Geometry check sheet. Reference: drawing and pictorial views, mm from the part's lowest x, y, z. A direction names the side the tool comes from. Give positions to 0.01 mm unless a question says otherwise; leave off trailing zeros. Write each loop counter-clockwise with the first axis right and the second up, starting at its lowest first coordinate (ties: lowest second). Pieces come first, ordered by that corner, then holes. Notation, with made-up numbers: (39.5, 41) -> (90.5, 41) arc R16 ccw to (90.5, 54) -> close; hole circle Ø9 at (26, -30). An arc over 180 degrees is marked (long way). Return JSON: item names as keys, results as strings.
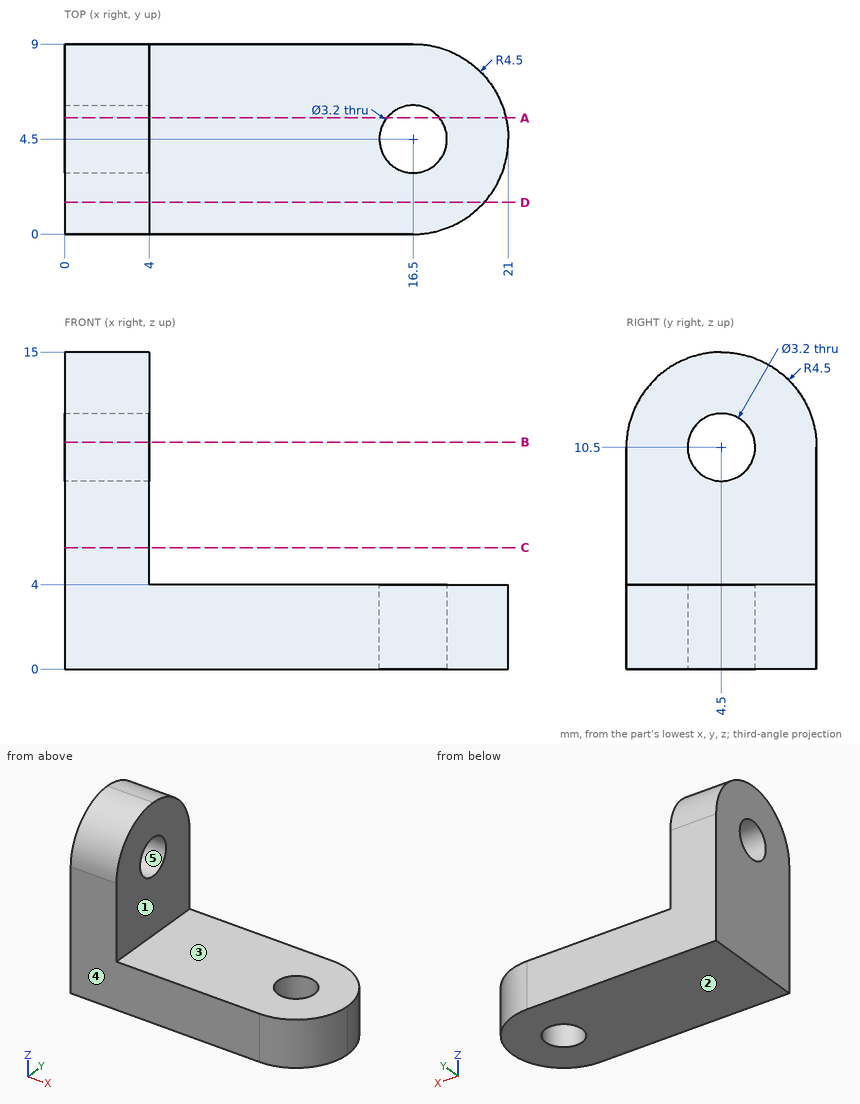
(1) Thickness scan on L1, parallel to Y at x = 2, z = 10.5; L2, parallel to X at y = 4.5, z = 1.45; L3, parallel to X at y = 1, z = 8. Record the ranges inside material, lowest first.
Reply:
{"L1": "0 to 2.9, 6.1 to 9", "L2": "0 to 14.9, 18.1 to 21", "L3": "0 to 4"}
(2) Cross-section at C-C on z = 5.75. Enter the section's corners in (x, y).
Reply:
{"outline": "(0, 0) -> (4, 0) -> (4, 9) -> (0, 9) -> close"}
(3) Cross-section at B-B on z = 10.75. Enter the section's corners in (x, y).
Reply:
{"outline": "(0, 0.01) -> (4, 0.01) -> (4, 2.92) -> (0, 2.92) -> close; (0, 6.08) -> (4, 6.08) -> (4, 8.99) -> (0, 8.99) -> close"}
(4) Set-up check for the marked faces 1 and 2: record each of +Z, -Z, +X, -X, +Y, -Y from which the full face is reachable in a straight line by a thin tool's end or side.
Reply:
{"face 1": "+Z, +X, +Y, -Y", "face 2": "-Z, +X, -X, +Y, -Y"}
(5) Cross-section at D-D on y = 1.5. Enter the section's corners in (x, z).
Reply:
{"outline": "(0, 0) -> (19.85, 0) -> (19.85, 4) -> (4, 4) -> (4, 13.85) -> (0, 13.85) -> close"}
(6) Depth check by flat-ended pin: pin 1 Ø1.5 at (x, z) = (11, 3) entering from -Y; pin 2 Ø3 at (y, z) = (4, 10.5) entering from +X; pin 3 Ø3 at (y, z) = (4.5, 10.5) entering from +X; pin 4 Ø2 at (x, y) = (12, 2) entering from +Z. Enter the tip coordinate at first touch or a pass-through.
Reply:
{"pin 1": "y = 0", "pin 2": "x = 4", "pin 3": "through", "pin 4": "z = 4"}
(7) Cross-section at A-A on y = 5.5. Enter the section's corners in (x, z), then the cut area to 3 significant figures.
Reply:
{"outline": "(0, 0) -> (15.25, 0) -> (15.25, 4) -> (4, 4) -> (4, 9.25) -> (0, 9.25) -> close; (0, 11.75) -> (4, 11.75) -> (4, 14.89) -> (0, 14.89) -> close; (17.75, 0) -> (20.89, 0) -> (20.89, 4) -> (17.75, 4) -> close", "area": "107 mm^2"}
(8) Release check for a two-part mould opening along Y. For the marked faces 3, 4 and 5 record: pulls with the +Y half, pulls with the -Y half, needs draft (parallel to the pull), parting line crosses it, or undercut.
Reply:
{"face 3": "needs draft", "face 4": "pulls with the -Y half", "face 5": "undercut"}
